from build123d import *

# Parameters (mm, degrees)
SKETCH_1_R      = 1
SKETCH_1_R_2    = 1.6
EXTRUDE_1_DEPTH = 1


with BuildPart() as part:
    # 草图1 → 凸台-拉伸1 (new body, symmetric)
    with BuildSketch(Plane.XY):
        with BuildLine():
            Line((0.874328329, 3.389033782), (-6.043528055, 5.173754207))
            ThreePointArc((-6.043528055, 5.173754207), (-8.518069078, 6.106819418), (-10.734845082, 7.548994201))
            ThreePointArc((-10.734845082, 7.548994201), (-12.857231055, 7.806973967), (-14, 6))
            Line((-14, 6), (-14, 1.110000054))
            Line((-14, 1.110000054), (-7.170013537, -2.005324011))
            ThreePointArc((-7.170013537, -2.005324011), (-6.317743639, -2.743301367), (-6, -3.824973007))
            Line((-6, -3.824973007), (-6, -14.200378782))
            Line((-6, -14.200378782), (-1.20605244, -14.456265808))
            ThreePointArc((-1.20605244, -14.456265808), (0.702747897, -15.147812467), (1.906524604, -16.782644918))
            Line((1.906524604, -16.782644918), (5.172173145, -26.001696201))
            ThreePointArc((5.172173145, -26.001696201), (8.931003799, -27.851882173), (10.874170567, -24.140265418))
            Line((10.874170567, -24.140265418), (3.353198995, 1.003023678))
            ThreePointArc((3.353198995, 1.003023678), (2.427191355, 2.521654641), (0.874328329, 3.389033782))
        make_face()
        with Locations((-12, 6)):
            Circle(SKETCH_1_R, mode=Mode.SUBTRACT)
        with Locations((8, -25)):
            Circle(SKETCH_1_R, mode=Mode.SUBTRACT)
        Circle(SKETCH_1_R_2, mode=Mode.SUBTRACT)
    extrude(amount=EXTRUDE_1_DEPTH, both=True)


solid = part.part
Design review of the part built by this model. Coordinates are the model's own, in mm. A direction names the side the tool comes from. Coordinates: 2 decimals unless noted, no trailing zeros. Loops run counter-clockwise (first coordinate to the right, second up) from the corner with the lowest first, then second, coordinate; pieces in that order, holes last. Notation, with made-up numbers: (-34.5, 69) -> (-2.5, 69) arc R24 cw to (-2.5, 107) -> close; hole circle Ø2 at (70.5, 1). An arc over 180 degrees is marked (long way). Use a Markdown table: item, result. Add a question column.
Item 1: We need section C-C, the plane y = -25. Write out the cut boundary in (x, z), and give its area (3 significant figures).
Item 2: Machinability: for faces 5 (the flat face through (-6, -9, 0)), 6 (the cylindrical face through (-1.27, -0.97, -0.01)), which of the approach directions +Z, -Z, +X, -X, +Y, -Y give a long, thin tool a straight path to every point of the face, cutting with its end or side? Answer none if there is none.
Item 3: Clearance check with flat-ended pins moving along their axes: P1, Ø0.6, axis at y = -7, z = 0, coming from the -X side; P2, Ø1, axis at y = -0.5, z = -0.5, coming from the -X side; P3, Ø1.6, axis at x = -12, y = 6, coming from the -Z side. State where each tip first meets the part, or that it passes through.
Item 4: We need section A-A, the plane z = 0.7. Write out the cut boundary in (x, y), and give its area (3 significant figures).
Item 5: The part is to be moulded in two halves that separate along X. For faces 1 (the cylindrical face through (8, -26, 0)), 2 (the cylindrical face through (-6.326, -2.73, 0.014)), 3 (the cylindrical face through (-12.83, 7.82, 0.01)), 4 (the cylindrical face through (2.45, 2.5, 0.01)), say which applies: +X half, -X half, draft (parallel to the pull), parting line (faces both ways), or undercut.
Item 6: We need section D-D, the plane y = -10. Write out the cut boundary in (x, z).
Item 7: We need section B-B, the plane x = 0. Write out the cut boundary in (y, z).
Item 8: Wall thickness on L1, parallel to Y at x = 0, z = 0.5; L2, parallel to Y at x = -11.25, z = 0.35; L3, parallel to Y at x = -6.75, z = -0.3: over which ranges is each line inside the solid? List them lowest first. Write a range as from..to.
Numbers:
| question | item | result |
|---|---|---|
| 1 | outline | (4.82, -1) -> (7, -1) -> (7, 1) -> (4.82, 1) -> close; (9, -1) -> (11, -1) -> (11, 1) -> (9, 1) -> close |
| 1 | area | 8.37 mm^2 |
| 2 | face 5 | +Z, -Z, -X, -Y |
| 2 | face 6 | +Z, -Z |
| 3 | P1 | stops at x = -6 |
| 3 | P2 | stops at x = -11.57 |
| 3 | P3 | passes through |
| 4 | outline | (-14, 1.11) -> (-7.17, -2.01) arc R2 cw to (-6, -3.82) -> (-6, -14.2) -> (-1.21, -14.46) arc R3.5 cw to (1.91, -16.78) -> (5.17, -26) arc R3 ccw to (10.87, -24.14) -> (3.35, 1) arc R3.5 ccw to (0.87, 3.39) -> (-6.04, 5.17) arc R12.26 cw to (-10.73, 7.55) arc R2 ccw to (-14, 6) -> close; hole circle Ø2 at (-12, 6); hole circle Ø3.2 at (0, 0); hole circle Ø2 at (8, -25) |
| 4 | area | 337 mm^2 |
| 5 | face 1 | undercut |
| 5 | face 2 | -X half |
| 5 | face 3 | parting line |
| 5 | face 4 | +X half |
| 6 | outline | (-6, -1) -> (6.64, -1) -> (6.64, 1) -> (-6, 1) -> close |
| 7 | outline | (-14.74, -1) -> (-1.6, -1) -> (-1.6, 1) -> (-14.74, 1) -> close; (1.6, -1) -> (3.61, -1) -> (3.61, 1) -> (1.6, 1) -> close |
| 8 | L1 | y = -14.74..-1.6, 1.6..3.61 |
| 8 | L2 | y = -0.14..5.34, 6.66..7.85 |
| 8 | L3 | y = -2.26..5.38 |
